Can you work these out from the model? Positions are in its coordinate system, mm. Give positions to 0.01 mm unless a question says otherwise; leave off trailing zeros. Order: outer loops, then holes, each group sorted by start corner. A loop starts at its lowest first (then second) coordinate and runs counter-clockwise, first axis right, second up. Notation, with made-up numbers: (-27, -29.75) - (0, -29.75) arc R15 ccw to (0, -17.75) - close; hole circle Ø9 at (85.5, 2). An arc over 180 degrees is marked (long way). Use one line per item in the form item = value. Start each with the question number.
1) Please list where these lines run through material, in increasing order: probe 1 along Y at (x, z) = (-33, 9); probe 2 along Y at (x, z) = (35, 15.5); probe 3 along X at (y, z) = (-247.5, -17).
2) Suppose I cut it at C-C, the plane x = -19.5. Write out the boundary of the cut face in (y, z), and give its area (3 significant figures).
3) For pin 1 (3 mm diameter, centred on x = -20, z = 1.5, fed in from -Y); pin 2 (10 mm diameter, centred on x = 20, z = -10, fed in from -Y), each with a flat end and sliding along its axis, tell me the tip position at first contact or that it passes through.
4) Suppose I cut it at B-B, the plane x = 16. Write out the boundary of the cut face in (y, z), and give its area (3 significant figures).
```python
from build123d import *

# Parameters (mm, degrees)
F0_W     = 88.9
F0_H     = 38.1
F1_DEPTH = 304.8
F2_SIZE2 = 88.89999
F2_SIZE  = 88.89999


# Not quite as in the source:
# - a fillet or chamfer is up to 0.001 mm smaller than in the source, because OpenCascade refuses the exact size


with BuildPart() as f1:
    # F0 (on Front) → F1 (new body, symmetric)
    with BuildSketch(Plane.XZ):
        Rectangle(F0_W, F0_H)
    extrude(amount=F1_DEPTH, both=True)

    # F2 (size 88.9 and 88.9 in the source; OpenCascade refuses exactly that, so slightly less here)
    f2_edges = [f1.edges().sort_by_distance(p)[0] for p in [
        (44.45, -304.8, 0),
    ]]
    chamfer(f2_edges, length=F2_SIZE, length2=F2_SIZE2)


solid = f1.part
```
Result sheet:
q1.probe_1 = -293.35 to 304.8
q1.probe_2 = -225.35 to 304.8
q1.probe_3 = -44.45 to 12.85
q2.outline = (-279.85, -19.05) - (304.8, -19.05) - (304.8, 19.05) - (-279.85, 19.05) - close
q2.area = 22,300 mm²
q3.pin_1 = -281.85
q3.pin_2 = -245.35
q4.outline = (-244.35, -19.05) - (304.8, -19.05) - (304.8, 19.05) - (-244.35, 19.05) - close
q4.area = 20,900 mm²
